```python
from build123d import *

# Parameters (mm, degrees)
SKETCH_1_W      = 15
SKETCH_1_H      = 10.2
SKETCH_1_W_2    = 3.5
SKETCH_1_H_2    = 11
EXTRUDE_1_DEPTH = 1.1
EXTRUDE_2_DEPTH = 0.9
SKETCH_3_W      = 0.4
SKETCH_3_H      = 12
EXTRUDE_3_DEPTH = 1
EXTRUDE_4_DEPTH = 1.5


with BuildPart() as part:
    # 草图1 → 凸台-拉伸1 (new body)
    with BuildSketch(Plane(origin=(0, 0, 0), x_dir=(1, 0, 0), z_dir=(0, 1, 0))):
        with BuildLine():
            Line((-0.7, 0.6), (-0.7, -10.8))
            Line((-0.7, -10.8), (15, -10.8))
            Line((15, -10.8), (15, -11.8))
            ThreePointArc((15, -11.8), (15.175735931, -12.224264069), (15.6, -12.4))
            Line((15.6, -12.4), (20.5, -12.4))
            Line((20.5, -12.4), (20.5, 2.2))
            Line((20.5, 2.2), (15.6, 2.2))
            ThreePointArc((15.6, 2.2), (15.175735931, 2.024264069), (15, 1.6))
            Line((15, 1.6), (15, 0.6))
            Line((15, 0.6), (-0.7, 0.6))
        make_face()
        with Locations((7.5, -5.1)):
            Rectangle(SKETCH_1_W, SKETCH_1_H, mode=Mode.SUBTRACT)
        with Locations((18.25, -5.1)):
            Rectangle(SKETCH_1_W_2, SKETCH_1_H_2, mode=Mode.SUBTRACT)
    extrude(amount=EXTRUDE_1_DEPTH)

    # 草图2 → 凸台-拉伸2 (add)
    with BuildSketch(Plane(origin=(0, 1.1, 0), x_dir=(1, 0, 0), z_dir=(0, 1, 0))):
        with BuildLine():
            Line((15, -10.8), (-0.7, -10.8))
            Line((-0.7, -10.8), (-0.7, 0.6))
            Line((-0.7, 0.6), (15, 0.6))
            Line((15, 0.6), (15, 1.6))
            ThreePointArc((15, 1.6), (15.175735931, 2.024264069), (15.6, 2.2))
            Line((15.6, 2.2), (20.5, 2.2))
            Line((20.5, 2.2), (20.5, -12.4))
            Line((20.5, -12.4), (15.6, -12.4))
            ThreePointArc((15.6, -12.4), (15.175735931, -12.224264069), (15, -11.8))
            Line((15, -11.8), (15, -10.8))
        make_face()
        Polygon((15, 0), (0, 0), (0, -10.2), (15, -10.2), (15, -8.9), (15.8, -8.9), (15.8, -10.8), (16.3, -11.3), (20, -11.3), (20, 1.1), (16.3, 1.1), (15.8, 0.6), (15.8, -1.3), (15, -1.3), align=None, mode=Mode.SUBTRACT)
    extrude(amount=EXTRUDE_2_DEPTH)

    # 草图3 → 凸台-拉伸3 (add)
    with BuildSketch(Plane.XZ):
        with BuildLine():
            Line((20.5, -2.2), (15.6, -2.2))
            ThreePointArc((15.6, -2.2), (15.175735931, -2.024264069), (15, -1.6))
            Line((15, -1.6), (15, 11.8))
            ThreePointArc((15, 11.8), (15.175735931, 12.224264069), (15.6, 12.4))
            Line((15.6, 12.4), (20.5, 12.4))
            Line((20.5, 12.4), (20.5, -2.2))
        make_face()
        with Locations((17.05, 5.1)):
            Rectangle(SKETCH_3_W, SKETCH_3_H, mode=Mode.SUBTRACT)
        with Locations((17.8, 5.1)):
            Rectangle(SKETCH_3_W, SKETCH_3_H, mode=Mode.SUBTRACT)
        with Locations((18.55, 5.1)):
            Rectangle(SKETCH_3_W, SKETCH_3_H, mode=Mode.SUBTRACT)
        with Locations((19.3, 5.1)):
            Rectangle(SKETCH_3_W, SKETCH_3_H, mode=Mode.SUBTRACT)
    extrude(amount=EXTRUDE_3_DEPTH)

    # 草图4 → 凸台-拉伸4 (add)
    with BuildSketch(Plane.ZY.offset(-15)):
        Polygon((11.8, 2), (11.8, -1), (-1.6, -1), (-1.6, 2), (-1.2, 2), (-1.2, -0.6), (11.4, -0.6), (11.4, 2), align=None)
    extrude(amount=EXTRUDE_4_DEPTH)


solid = part.part
```
Can you work these out from the model? Positions are in its coordinate system, mm. A direction names the side the tool comes from. Round coordinates to 2 decimals unless told otherwise and drop trailing zeros. Loops run counter-clockwise (first coordinate to the right, second up) from the corner with the lowest first, then second, coordinate; pieces in that order, holes last.
Item 1: Please list where these lines run through material, in increasing order: L1, parallel to X at y = 0.95, z = 6.25; L2, parallel to X at y = -0.4, z = 5; L3, parallel to X at y = -0.7, z = 5.25.
Item 2: Suppose I cut it at B-B, the plane x = 9.75. Write out the boundary of the cut face in (y, z), then the cut area to 3 significant figures.
Item 3: Suppose I cut it at A-A, the plane z = 4.25. State how many separate pieces and enclosed holes the cut face has, then the cut area to 3 significant figures.
Item 4: Suppose I cut it at D-D, the plane x = 14.75. Write out the boundary of the cut face in (y, z).
Item 5: Will these pins go through, and if not, where does the flat tip stop? pin 1 Ø1.5 at (x, z) = (10, 2.5) entering from +Y; pin 2 Ø0.6 at (x, y) = (9, 1) entering from -Z; pin 3 Ø0.8 at (y, z) = (-0.5, 7.5) entering from -X.
Item 6: Suppose I cut it at C-C, the plane y = 0.6. Write out the boundary of the cut face in (x, z).
Item 7: Which directions (+Z, -Z, +X, -X, +Y, -Y) give clear straight access to the entire face, cutting with the end or side of a thin tool? Please do faces 4 (the flat face through (15.4, 1.5, 1.3)), 5 (the flat face through (14, 1, -1.2)), 6 (the flat face through (14, 1, 11.8)).
Item 8: If we mould it in two halves opening along Z, with no side actions, what happens to faces 1 (the flat face through (-0.7, 1, 5)), 2 (the flat face through (18, 1, 12.4)), 3 (the flat face through (7, 1, 10.2))? For each: +Z half, -Z half, draft (parallel to the pull), parting line (faces both ways), or undercut.
Reported:
1. L1: x = -0.7 to 0, 15 to 16.5, 20 to 20.5
1. L2: x = 15 to 16.85, 17.25 to 17.6, 18 to 18.35, 18.75 to 19.1, 19.5 to 20.5
1. L3: x = 13.5 to 16.85, 17.25 to 17.6, 18 to 18.35, 18.75 to 19.1, 19.5 to 20.5
2. outline: (0, -0.6) - (2, -0.6) - (2, 0) - (0, 0) - close; (0, 10.2) - (2, 10.2) - (2, 10.8) - (0, 10.8) - close
2. area: 2.40 mm2
3. separate pieces: 6
3. enclosed holes: 0
3. area: 8.55 mm2
4. outline: (-1, -1.6) - (2, -1.6) - (2, -1.2) - (-0.6, -1.2) - (-0.6, 11.4) - (2, 11.4) - (2, 11.8) - (-1, 11.8) - close; (0, -0.6) - (2, -0.6) - (2, 0) - (0, 0) - close; (0, 10.2) - (2, 10.2) - (2, 10.8) - (0, 10.8) - close
5. pin 1: passes through
5. pin 2: stops at z = -0.6
5. pin 3: stops at x = 13.5
6. outline: (-0.7, -0.6) - (15, -0.6) - (15, -1.2) - (13.5, -1.2) - (13.5, -1.6) - (15, -1.6) arc R0.6 ccw to (15.6, -2.2) - (20.5, -2.2) - (20.5, 12.4) - (15.6, 12.4) arc R0.6 ccw to (15, 11.8) - (13.5, 11.8) - (13.5, 11.4) - (15, 11.4) - (15, 10.8) - (-0.7, 10.8) - close; hole (0, 0) - (15, 0) - (15, 10.2) - (0, 10.2) - close; hole (16.5, -0.4) - (20, -0.4) - (20, 10.6) - (16.5, 10.6) - close
7. face 4: +Y
7. face 5: -X, +Y
7. face 6: +Z, -X, +Y, -Y
8. face 1: draft
8. face 2: +Z half
8. face 3: undercut
